Geometry check sheet. Reference: drawing and pictorial views, mm from the part's lowest x, y, z. A direction names the side the tool comes from. Round coordinates to 2 decimals unless told otherwise and drop trailing zeros. Order: outer loops, then holes, each group sorted by start corner. A loop starts at its lowest first (then second) coordinate and runs counter-clockwise, first axis right, second up.
(1) Cross-section at C-C on z = 11. Enter the section's corners in (x, y).
(2) Cross-section at D-D on y = 7.25. Enter the section's corners in (x, z), and give its area (3 significant figures).
(3) Set-up check for the marked faces 4, 5 and 6: record each of +Z, -Z, +X, -X, +Y, -Y from which the full face is reachable in a straight line by a thin tool's end or side.
(4) Gauge pin test, flat ends, axial feed: P1, Ø5, axis at x = 3.7, y = 2.95, coming from the -Z side; P2, Ø3, axis at x = 15, y = 9.25, coming from the -Z side; P3, Ø4, axis at x = 17.5, y = 10, coming from the +Z side; P4, Ø6, axis at x = 10.5, y = 15, coming from the -Z side. Record the tip position at first contact, or that the pin passes through.
(5) Thickness scan on L1, parallel to Y at x = 5.75, z = 9.5; L2, parallel to X at y = 12.75, z = 10; L3, parallel to X at y = 9.25, z = 3. Record the ranges inside material, lowest first.
(6) Cross-section at A-A on y = 9.25. Enter the section's corners in (x, z), and give its area (3 significant figures).
(7) Cross-section at B-B on z = 8.5. Enter the section's corners in (x, y), and give its area (3 significant figures).
(8) Draft check along X on the marked faces 1, 2 and 3. Enter one of: pulls with the +X half, pulls with the -X half, needs draft (parallel to the pull), parting line crosses it, or undercut.
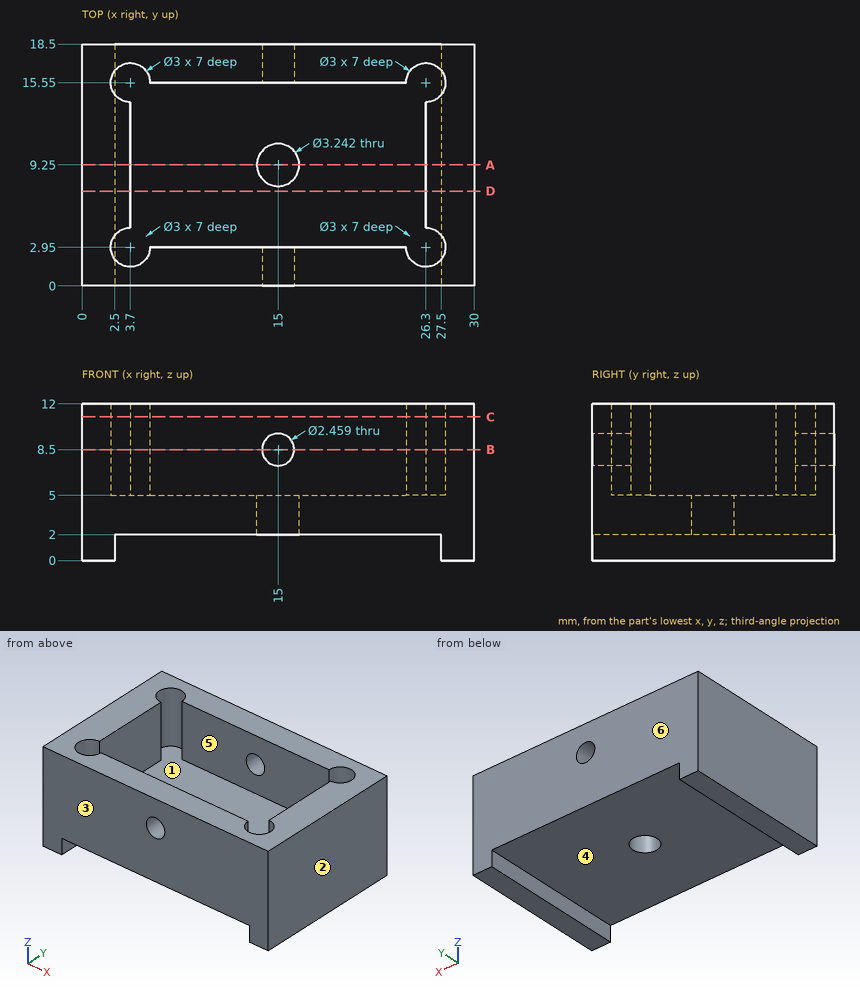
Found:
1. outline: (0, 0) - (30, 0) - (30, 18.5) - (0, 18.5) - close; hole (3.7, 4.45) arc R1.5 ccw (long way) to (5.2, 2.95) - (24.8, 2.95) arc R1.5 ccw (long way) to (26.3, 4.45) - (26.3, 14.05) arc R1.5 ccw (long way) to (24.8, 15.55) - (5.2, 15.55) arc R1.5 ccw (long way) to (3.7, 14.05) - close
2. outline: (0, 0) - (2.5, 0) - (2.5, 2) - (27.5, 2) - (27.5, 0) - (30, 0) - (30, 12) - (26.3, 12) - (26.3, 5) - (3.7, 5) - (3.7, 12) - (0, 12) - close
2. area: 152 mm2
3. face 4: -Z, +Y, -Y
3. face 5: +Z
3. face 6: +Z, -Z, +X, -X, +Y
4. P1: stops at z = 0
4. P2: passes through
4. P3: stops at z = 5
4. P4: stops at z = 2
5. L1: y = 0 to 2.95, 15.55 to 18.5
5. L2: x = 0 to 3.7, 26.3 to 30
5. L3: x = 0 to 13.38, 16.62 to 30
6. outline: (0, 0) - (2.5, 0) - (2.5, 2) - (13.38, 2) - (13.38, 5) - (3.7, 5) - (3.7, 12) - (0, 12) - close; (16.62, 2) - (27.5, 2) - (27.5, 0) - (30, 0) - (30, 12) - (26.3, 12) - (26.3, 5) - (16.62, 5) - close
6. area: 142 mm2
7. outline: (0, 0) - (13.77, 0) - (13.77, 2.95) - (5.2, 2.95) arc R1.5 cw (long way) to (3.7, 4.45) - (3.7, 14.05) arc R1.5 cw (long way) to (5.2, 15.55) - (13.77, 15.55) - (13.77, 18.5) - (0, 18.5) - close; (16.23, 0) - (30, 0) - (30, 18.5) - (16.23, 18.5) - (16.23, 15.55) - (24.8, 15.55) arc R1.5 cw (long way) to (26.3, 14.05) - (26.3, 4.45) arc R1.5 cw (long way) to (24.8, 2.95) - (16.23, 2.95) - close
7. area: 235 mm2
8. face 1: undercut
8. face 2: pulls with the +X half
8. face 3: needs draft
